Work out the finished part from the listing and answer in its coordinate system (mm). A direction names the side the tool comes from. Give positions to 0.01 mm unless a question says otherwise; leave off trailing zeros. Loops run counter-clockwise (first coordinate to the right, second up) from the corner with the lowest first, then second, coordinate; pieces in that order, holes last. Notation, with made-up numbers: (57.5, 10.5) - (108.5, 10.5) arc R22 ccw to (108.5, 17.5) - close; hole circle Ø1 at (5, 64). An arc over 180 degrees is marked (long way). Use CSV: the item, a comma, the result in double quotes.
Autodesk Inventor part; units mm, degrees
ref_plane "YZ Plane" through (0, 0, 0) normal (1, 0, 0) x (0, 1, 0)
ref_plane "XZ Plane" through (0, 0, 0) normal (0, 1, 0) x (-1, 0, 0)
ref_plane "XY Plane" through (0, 0, 0) normal (0, 0, 1) x (1, 0, 0)
sketch "スケッチ1" plane through (0, 0, 0) normal (0, 1, 0) x (-1, 0, 0)
  line L0 (7.5, 8) -> (-7.5, 8)
  line L1 (-7.5, 8) -> (-7.5, -8)
  line L2 (-7.5, -8) -> (7.5, -8)
  line L3 (7.5, -8) -> (7.5, 8)
  line L4 (7.5, 8) -> (-7.5, -8) construction
  line L5 (-7.5, 8) -> (7.5, -8) construction
  line L6 (5.05, 2.05) -> (-5.05, 2.05)
  line L7 (-5.05, 2.05) -> (-5.05, -2.05)
  line L8 (-5.05, -2.05) -> (5.05, -2.05)
  line L9 (5.05, -2.05) -> (5.05, 2.05)
  line L10 (5.05, 2.05) -> (-5.05, -2.05) construction
  line L11 (-5.05, 2.05) -> (5.05, -2.05) construction
  point P0 (0, 0)
  dimension "d0" = 15
  dimension "d1" = 16
  dimension "d2" = 10.1
  dimension "d3" = 4.1
extrude "押し出し1" add sketch "スケッチ1" along normal blind 2
sketch "スケッチ2" plane through (0, 2, 0) normal (0, 1, 0) x (1, 0, 0)
  line L0 (-5.05, 2.05) -> (5.05, 2.05)
  line L1 (-5.05, 2.05) -> (5.05, 2.05)
  line L2 (5.05, 2.05) -> (5.05, 4.05)
  line L3 (5.05, 4.05) -> (-5.05, 4.05)
  line L4 (-5.05, 4.05) -> (-5.05, 2.05)
  line L5 (5.05, -2.05) -> (-5.05, -2.05)
  line L6 (-5.05, -2.05) -> (5.05, -2.05)
  line L7 (5.05, -2.05) -> (5.05, -4.05)
  line L8 (5.05, -4.05) -> (-5.05, -4.05)
  line L9 (-5.05, -4.05) -> (-5.05, -2.05)
  point P0 (0, 0)
  point P1 (5.05, 2.05)
  dimension "d6" = 2
  dimension "d7" = 2
extrude "押し出し2" add sketch "スケッチ2" along normal blind 7
fillet "フィレット1" radius 1 6 edges at (5.05, 2, 3.05) (0, 2, 4.05) (-5.05, 2, 3.05) (-5.05, 2, -3.05) (0, 2, -4.05) (5.05, 2, -3.05)
fillet "フィレット2" radius 2 4 edges at (7.5, 1, -8) (-7.5, 1, -8) (-7.5, 1, 8) (7.5, 1, 8)
equation "\"d7\" = d6"
properties part number "LRA_case1"
Item 1: A cutting plane is placed at C-C on x = -1. Determine the outline of the cut face in (y, z), and give its area (3 significant figures).
Determined:
outline,"(0, -8) - (2, -8) - (2, -5.05) arc R1 cw to (3, -4.05) - (9, -4.05) - (9, -2.05) - (0, -2.05) - close; (0, 2.05) - (9, 2.05) - (9, 4.05) - (3, 4.05) arc R1 cw to (2, 5.05) - (2, 8) - (0, 8) - close"
area,"52.2 mm²"
Item 2: Find the intervals of material crossed by line 1 (X direction, y = 1.5, z = -0.75); line 2 (Z direction, x = 5, y = 7); line 3 (Y direction, x = 0, z = 4.75), in increasing order.
Determined:
line 1,"x = -7.5 to -5.05, 5.05 to 7.5"
line 2,"z = -4.05 to -2.05, 2.05 to 4.05"
line 3,"y = 0 to 2.05"
Item 3: For faces 1 (the flat face through (0, 9, -3)), 2 (the flat face through (-5.05, 6, -3)), 3 (the flat face through (5.05, 6, -3)), 4 (the flat face through (5.05, 1, 0)), 5 (the flat face through (-7.5, 1, 0)), determine the directions among +Z, -Z, +X, -X, +Y, -Y from which every point of the face is accessible in a straight line to the end or side of a thin tool.
Determined:
face 1,"+Z, -Z, +X, -X, +Y"
face 2,"+Z, -Z, -X, +Y"
face 3,"+Z, -Z, +X, +Y"
face 4,"+Y, -Y"
face 5,"+Z, -Z, -X, +Y, -Y"
Item 4: A cutting plane is placed at D-D on y = 1.5. Determine the outline of the cut face in (x, z), and give its area (3 significant figures).
Determined:
outline,"(-7.5, -6) arc R2 ccw to (-5.5, -8) - (5.5, -8) arc R2 ccw to (7.5, -6) - (7.5, 6) arc R2 ccw to (5.5, 8) - (-5.5, 8) arc R2 ccw to (-7.5, 6) - close; hole (-5.05, -2.05) - (5.05, -2.05) - (5.05, 2.05) - (-5.05, 2.05) - close"
area,"195 mm²"
Item 5: A cutting plane is placed at B-B on z = 1. Determine the outline of the cut face in (x, y), and give its area (3 significant figures).
Determined:
outline,"(-7.5, 0) - (-5.05, 0) - (-5.05, 2) - (-7.5, 2) - close; (5.05, 0) - (7.5, 0) - (7.5, 2) - (5.05, 2) - close"
area,"9.80 mm²"
Item 6: The mould has two halves that part along X. Classify faces 6 (the flat face through (0, 1, -8)), 7 (the flat face through (-5.05, 6, 3)), 8 (the flat face through (-5.05, 1, 0)): pulls with the +X half, pulls with the -X half, needs draft (parallel to the pull), parting line crosses it, or undercut.
Determined:
face 6,"needs draft"
face 7,"pulls with the -X half"
face 8,"undercut"
Item 7: A cutting plane is placed at A-A on y = 7.5. Determine the outline of the cut face in (x, z), and give its area (3 significant figures).
Determined:
outline,"(-5.05, -4.05) - (5.05, -4.05) - (5.05, -2.05) - (-5.05, -2.05) - close; (-5.05, 2.05) - (5.05, 2.05) - (5.05, 4.05) - (-5.05, 4.05) - close"
area,"40.4 mm²"
Item 8: Given P1, Ø2, axis at y = 6.5, z = -3.5, coming from the +X side; P2, Ø1, axis at y = 5.5, z = 3, coming from the -X side; P3, Ø4.5, axis at x = -1.5, y = 5.5, coming from the -Z side; P4, Ø4, axis at x = 5, z = -3.5, coming from the -Y side, each flat-ended and moving along its own axis, determine where each tip first touches the part or whether it passes through.
Determined:
P1,"stops at x = 5.05"
P2,"stops at x = -5.05"
P3,"stops at z = -4.05"
P4,"stops at y = 0"
